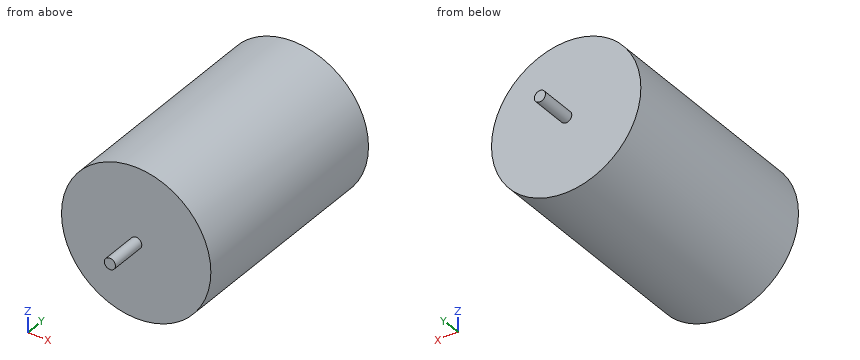
from build123d import *

# Parameters (mm, degrees)
F0_R      = 25.4
F1_DEPTH  = 38.1
F1_FACE_R = 25.4
F2_DEPTH  = 38.1
F4_R      = 1.905
F5_DEPTH  = 12.7
F3_R      = 1.905
F6_DEPTH  = 12.7


with BuildPart() as f1:
    # F0 (on Front) → F1 (new body)
    with BuildSketch(Plane.XZ):
        Circle(F0_R)
    extrude(amount=F1_DEPTH)

    # F1_face (on face) → F2 (join)
    with BuildSketch(Plane(origin=(0, 0, 0), x_dir=(1, 0, 0), z_dir=(0, 1, 0))):
        Circle(F1_FACE_R)
    extrude(amount=F2_DEPTH)

    # F4 (on face) → F5 (join)
    with BuildSketch(Plane(origin=(0, 38.1, 0), x_dir=(-1, 0, 0), z_dir=(0, 1, 0))):
        Circle(F4_R)
    extrude(amount=F5_DEPTH)

    # F3 (on face) → F6 (join)
    with BuildSketch(Plane.XZ.offset(38.1)):
        Circle(F3_R)
    extrude(amount=F6_DEPTH)


solid = f1.part
Could you check a few things on this model? Use its own coordinates, in mm. Round coordinates to 2 decimals unless told otherwise and drop trailing zeros. Order: outer loops, then holes, each group sorted by start corner. A loop starts at its lowest first (then second) coordinate and runs counter-clockwise, first axis right, second up.
Q1. I'm going to push flat-ended pins straight in: P1, Ø3, axis at x = -7, y = 29, coming from the +Z side; P2, Ø5, axis at x = -11, z = 6.5, coming from the +Y side; P3, Ø5, axis at x = 16, z = 13.5, coming from the -Y side; P4, Ø1, axis at y = -40.5, z = 8, coming from the +X side. Where does each tip first touch, or does it pass through?
Geometry says:
P1: stops at z = 24.8
P2: stops at y = 38.1
P3: stops at y = -38.1
P4: passes through
Q2. Imagine slicing it at C-C, the plane y = 1.5. List the corners of the cut face in (x, z) for me, then the cut area to 3 significant figures.
Geometry says:
outline: circle Ø50.8 at (0, 0)
area: 2,030 mm2
Q3. Imagine slicing it at D-D, the plane z = 22.5. List the corners of the cut face in (x, y) for me, then the cut area to 3 significant figures.
Geometry says:
outline: (-11.79, -38.1) - (11.79, -38.1) - (11.79, 38.1) - (-11.79, 38.1) - close
area: 1,800 mm2
Q4. Imagine slicing it at B-B, the plane x = 0. List the corners of the cut face in (y, z) for me (3 decimals).
Geometry says:
outline: (-50.8, -1.905) - (-38.1, -1.905) - (-38.1, -25.4) - (38.1, -25.4) - (38.1, -1.905) - (50.8, -1.905) - (50.8, 1.905) - (38.1, 1.905) - (38.1, 25.4) - (-38.1, 25.4) - (-38.1, 1.905) - (-50.8, 1.905) - close
Q5. Please list where these lines run through material, in increasing order: probe 1 along Y at (x, z) = (-14, -17); probe 2 along Z at (x, y) = (6, -29.5); probe 3 along X at (y, z) = (25, 6.5).
Geometry says:
probe 1: y = -38.1 to 38.1
probe 2: z = -24.68 to 24.68
probe 3: x = -24.55 to 24.55
Q6. Imagine slicing it at A-A, the plane z = 0. List the corners of the cut face in (x, y) for me (3 decimals), then the cut area to 3 significant figures.
Geometry says:
outline: (-25.4, -38.1) - (-1.905, -38.1) - (-1.905, -50.8) - (1.905, -50.8) - (1.905, -38.1) - (25.4, -38.1) - (25.4, 38.1) - (1.905, 38.1) - (1.905, 50.8) - (-1.905, 50.8) - (-1.905, 38.1) - (-25.4, 38.1) - close
area: 3,970 mm2
